Geometry: see drawing. Coordinates: mm, zero at the bounding-box minimum. A direction names the side the tool comes from. Round coordinates to 2 decimals unless told otherwise and drop trailing zeros. Loops run counter-clockwise (first coordinate to the right, second up) from the corner with the lowest first, then second, coordinate; pieces in that order, holes last. Notation, with made-up numbers: (81, 69) - (98, 69) arc R21 ccw to (98, 93) - close; hole circle Ø1 at (25, -36.5). An arc over 180 degrees is marked (long way). Write item = value, one per line. Start each with the question number.
Item 1: Access query for the marked faces 1, 2, 3 and 4. Directions: +Z, -Z, +X, -X, +Y, -Y. A direction counts if a zero-diameter tool reaches every point of the face in a straight line with its end or side. Return the directions, or none.
Item 2: Line query: line 1 (Y direction, x = 26.4, z = 20.7); line 2 (X direction, y = 19, z = 51.5); line 3 (Y direction, x = 40.05, z = 56.2) (1 decimal). Output: solid intervals per line, ascending. Write a range as from..to.
Item 3: First-contact query: pin 1 (4.5 mm diameter, centred on x = 22.5, y = 46, fed in from -Z); pin 2 (4 mm diameter, centred on y = 69, z = 8, fed in from +X); pin 3 (5 mm diameter, centred on x = 20, z = 23, fed in from -Y). Flat tips, straight axial feed; report the tip coordinate or a pass-through.
Item 4: Draft query along X for the marked faces 5, 6 and 7. Return one class per face: pulls with the +X half, pulls with the -X half, needs draft (parallel to the pull), parting line crosses it, or undercut.
Item 5: Section A-A (y = 93.5). Return loops of the section in (x, z).
Item 6: Section C-C (y = 63). Return loops of the section in (x, z).
Item 7: Section D-D (z = 55). Return loops of the section in (x, y).
Item 8: Section B-B (x = 26.4). Return loops of the section in (y, z), plus the area to 3 significant figures.
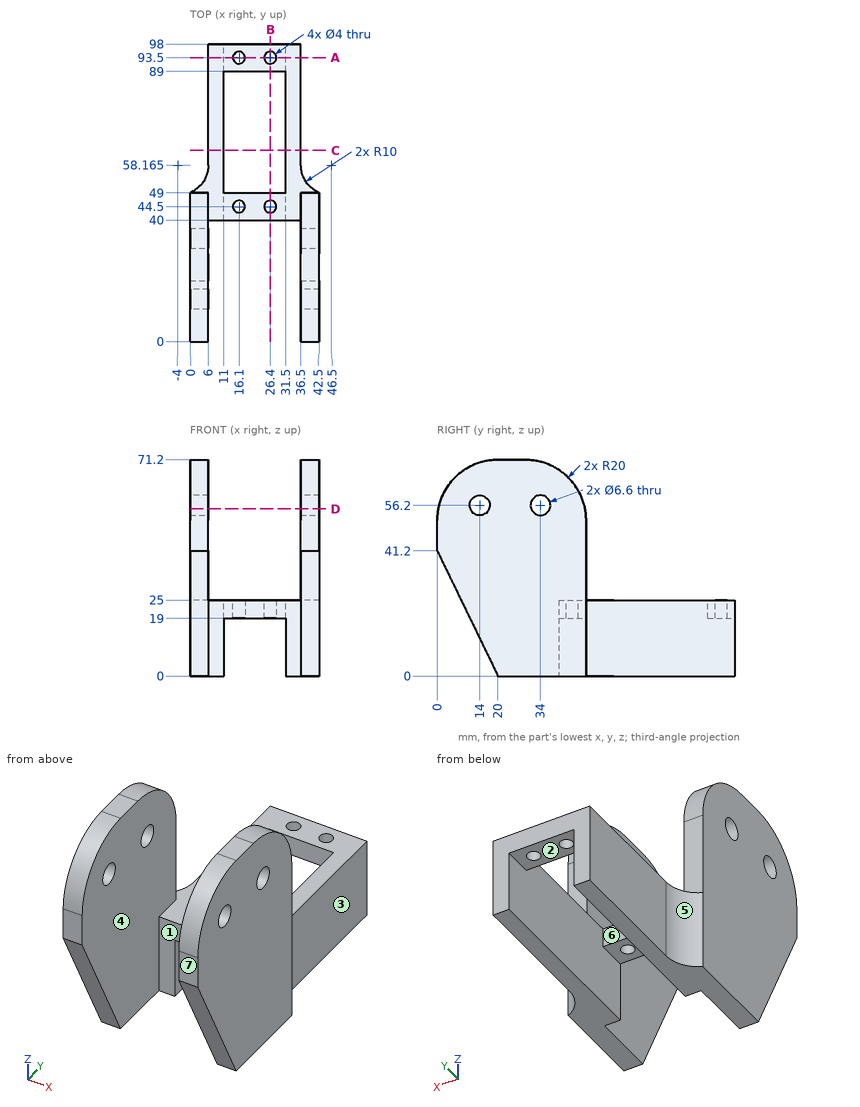
Taken from the geometry:
q1.face_1 = +Z, -Z, -Y
q1.face_2 = -Z, +Y, -Y
q1.face_3 = +Z, -Z, +X, +Y
q1.face_4 = +Z, -Y
q2.line_1 = 40..42.5, 46.5..49, 89..91.5, 95.5..98
q2.line_2 = 0..6, 36.5..42.5
q2.line_3 = 0.6..10.7, 17.3..30.7, 37.3..48.4
q3.pin_1 = 19
q3.pin_2 = 36.5
q3.pin_3 = 40
q4.face_5 = pulls with the -X half
q4.face_6 = undercut
q4.face_7 = needs draft
q5.outline = (6, 0) - (11, 0) - (11, 19) - (14.1, 19) - (14.1, 25) - (6, 25) - close; (18.1, 19) - (24.4, 19) - (24.4, 25) - (18.1, 25) - close; (28.4, 19) - (31.5, 19) - (31.5, 0) - (36.5, 0) - (36.5, 25) - (28.4, 25) - close
q6.outline = (6, 0) - (11, 0) - (11, 25) - (6, 25) - close; (31.5, 0) - (36.5, 0) - (36.5, 25) - (31.5, 25) - close
q7.outline = (0, 0.36) - (6, 0.36) - (6, 10.93) - (0, 10.93) - close; (0, 17.07) - (6, 17.07) - (6, 30.93) - (0, 30.93) - close; (0, 37.07) - (6, 37.07) - (6, 48.64) - (0, 48.64) - close; (36.5, 0.36) - (42.5, 0.36) - (42.5, 10.93) - (36.5, 10.93) - close; (36.5, 17.07) - (42.5, 17.07) - (42.5, 30.93) - (36.5, 30.93) - close; (36.5, 37.07) - (42.5, 37.07) - (42.5, 48.64) - (36.5, 48.64) - close
q8.outline = (40, 19) - (42.5, 19) - (42.5, 25) - (40, 25) - close; (46.5, 19) - (49, 19) - (49, 25) - (46.5, 25) - close; (89, 19) - (91.5, 19) - (91.5, 25) - (89, 25) - close; (95.5, 19) - (98, 19) - (98, 25) - (95.5, 25) - close
q8.area = 60.0 mm^2
